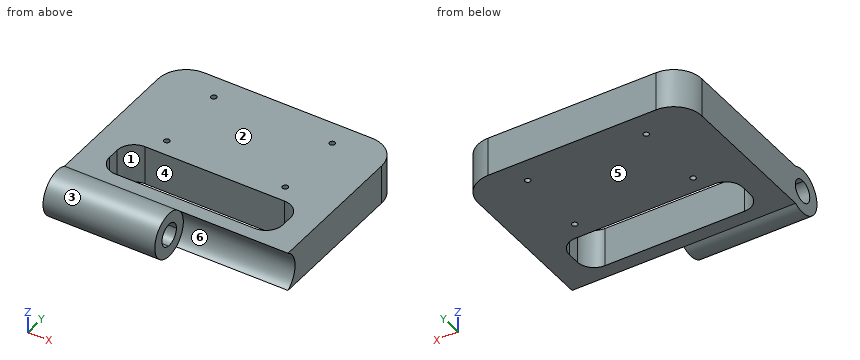
```python
from build123d import *

# Parameters (mm, degrees)
SKETCH1_W                = 40
SKETCH1_H                = 33.082043622
BOSS_EXTRUDE1_DEPTH      = 7
SKETCH2_R                = 4.1
CUT_EXTRUDE1_DEPTH       = 20
BOSS_EXTRUDE2_DEPTH      = 11
BOSS_EXTRUDE2_DEPTH_BACK = 9
SKETCH3_R                = 4
SKETCH3_R_2              = 2
FILLET1_R                = 5
SKETCH4_R                = 0.5
SKETCH4_W                = 31
SKETCH4_H                = 8.146627971
CUT_EXTRUDE2_DEPTH       = 45.095541639
FILLET2_R                = 3
SKETCH5_R                = 2
CUT_EXTRUDE3_DEPTH       = 56.229329833


with BuildPart() as part:
    # Sketch1 → Boss-Extrude1 (new body)
    with BuildSketch(Plane.XY):
        with Locations((-2.229213179, -16.994598242)):
            Rectangle(SKETCH1_W, SKETCH1_H)
    extrude(amount=BOSS_EXTRUDE1_DEPTH)

    # Sketch2 → Cut-Extrude1 (cut)
    with BuildSketch(Plane(origin=(17.770786821, 0, 0), x_dir=(0, 0, -1), z_dir=(1, 0, 0))):
        with Locations((-3.5, -33.535620053)):
            Circle(SKETCH2_R)
    extrude(amount=-CUT_EXTRUDE1_DEPTH, mode=Mode.SUBTRACT)

    # Sketch3 → Boss-Extrude2 (add, two sides: drawn at the far end of the back side and taken through both)
    with BuildSketch(Plane(origin=(-13.229213179, 0, 0), x_dir=(0, 0, -1), z_dir=(1, 0, 0)).offset(-BOSS_EXTRUDE2_DEPTH_BACK)):
        with Locations((-3.5, -33.336696075)):
            Circle(SKETCH3_R)
        with Locations((-3.5, -33.336696075)):
            Circle(SKETCH3_R_2, mode=Mode.SUBTRACT)
    extrude(amount=BOSS_EXTRUDE2_DEPTH + BOSS_EXTRUDE2_DEPTH_BACK)

    # Fillet1
    fillet1_edges = [part.edges().sort_by_distance(p)[0] for p in [
        (-22.229213179, -0.453576431, 3.5),
        (17.770786821, -0.453576431, 3.5),
    ]]
    fillet(fillet1_edges, radius=FILLET1_R)

    # Sketch4 → Cut-Extrude2 (cut, through all)
    with BuildSketch(Plane(origin=(0, 0, 0), x_dir=(-1, 0, 0), z_dir=(0, 0, -1))):
        with Locations((-8.470786821, -4.753576431)):
            Circle(SKETCH4_R)
        with Locations((12.729213179, -4.753576431)):
            Circle(SKETCH4_R)
        with Locations((12.729213179, -17.753576431)):
            Circle(SKETCH4_R)
        with Locations((-8.470786821, -17.753576431)):
            Circle(SKETCH4_R)
        with Locations((2.229213179, -24.826890417)):
            Rectangle(SKETCH4_W, SKETCH4_H)
    extrude(amount=-CUT_EXTRUDE2_DEPTH, mode=Mode.SUBTRACT)

    # Fillet2
    fillet2_edges = [part.edges().sort_by_distance(p)[0] for p in [
        (-17.729213179, -20.753576431, 3.5),
        (-17.729213179, -28.900204402, 3.5),
        (13.270786821, -28.900204402, 3.5),
        (13.270786821, -20.753576431, 3.5),
    ]]
    fillet(fillet2_edges, radius=FILLET2_R)

    # Sketch5 → Cut-Extrude3 (cut, through all)
    with BuildSketch(Plane.ZY.offset(22.229213179)):
        with Locations(Location((3.5, -33.336696075, 0), (0, 0, 90))):
            Circle(SKETCH5_R)
    extrude(amount=-CUT_EXTRUDE3_DEPTH, mode=Mode.SUBTRACT)


solid = part.part
```
The model under review builds one solid part; all positions refer to its coordinate system, in mm. Face numbers are marked on the shaded views. A direction names the side the tool comes from. Give positions to 0.01 mm unless a question says otherwise; leave off trailing zeros. Order: outer loops, then holes, each group sorted by start corner. A loop starts at its lowest first (then second) coordinate and runs counter-clockwise, first axis right, second up. Notation, with made-up numbers: (85, 27.25) - (89, 27.25) arc R23 cw to (89, 60.25) - close; hole circle Ø3 at (7.25, 26). An arc over 180 degrees is marked (long way). Use CSV: the item, a comma, the result in double quotes. Start each with the question number.
Q1. Clearance check with flat-ended pins moving along their axes: pin 1 Ø4 at (x, y) = (10.5, -32.5) entering from -Z; pin 2 Ø1.5 at (x, y) = (8.5, -12) entering from +Z; pin 3 Ø2 at (x, z) = (-1, 3) entering from -Y. State where each tip first meets the part, or that it passes through.
Q2. Tool access review of the marked faces 4, 5 and 6: name each direction out of +Z, -Z, +X, -X, +Y, -Y from which nothing blocks a thin tool from reaching the whole face with its end or side.
Q3. To check wall thickness, follow line 1 along Y through (x, z) = (6, 3.75); line 2 along X through (y, z) = (-24, 3.75); line 3 along Y through (x, z) = (-3.5, 2). State the ranges of each line that lie inside material, in increasing order. Write a range as [from, to].
Q4. The part is to be moulded in two halves that separate along Y. For the marked faces 1, 2 and 3, say which applies: +Y half, -Y half, draft (parallel to the pull), parting line (faces both ways), or undercut.
Q5. We need section A-A, the plane x = 0. Write out the cut boundary in (y, z).
Q6. We need section D-D, the plane y = -6. Write out the cut boundary in (x, z), and give its area (3 significant figures).
Q7. We need section B-B, the plane z = 4.75. Write out the cut boundary in (x, y), and give its area (3 significant figures).
Q8. We need section C-C, the plane x = -11.5. Write out the cut boundary in (y, z), and give its area (3 significant figures).
Outcome:
1,pin 1,"stops at z = 0"
1,pin 2,"stops at z = 7"
1,pin 3,"stops at y = -29.72"
2,face 4,"+Z, -Z"
2,face 5,"-Z, +X, -X, +Y"
2,face 6,"+X, -Y"
3,line 1,"y = [-29.44, -28.9], [-20.75, -0.45]"
3,line 2,"x = [-22.23, -17.73], [13.27, 17.77]"
3,line 3,"y = [-37.04, -34.66], [-32.01, -28.9], [-20.75, -0.45]"
4,face 1,"undercut"
4,face 2,"draft"
4,face 3,"parting line"
5,outline,"(-31.4, 0) - (-28.9, 0) - (-28.9, 7) - (-31.4, 7) arc R4.1 cw to start; (-20.75, 0) - (-0.45, 0) - (-0.45, 7) - (-20.75, 7) - close"
6,outline,"(-22.23, 0) - (17.77, 0) - (17.77, 7) - (-22.23, 7) - close"
6,area,"280 mm^2"
7,outline,"(-22.23, -37.14) - (-2.23, -37.14) - (-2.23, -34.9) - (-22.23, -34.9) - close; (-22.23, -31.78) - (-2.23, -31.78) - (-2.23, -29.63) - (17.77, -29.63) - (17.77, -5.45) arc R5 ccw to (12.77, -0.45) - (-17.23, -0.45) arc R5 ccw to (-22.23, -5.45) - close; hole (-17.73, -25.9) arc R3 ccw to (-14.73, -28.9) - (10.27, -28.9) arc R3 ccw to (13.27, -25.9) - (13.27, -23.75) arc R3 ccw to (10.27, -20.75) - (-14.73, -20.75) arc R3 ccw to (-17.73, -23.75) - close; hole circle Ø1 at (-12.73, -17.75); hole circle Ø1 at (-12.73, -4.75); hole circle Ø1 at (8.47, -17.75); hole circle Ø1 at (8.47, -4.75)"
7,area,"996 mm^2"
8,outline,"(-31.4, 0) - (-28.9, 0) - (-28.9, 7) - (-31.4, 7) arc R4 ccw (long way) to start; (-20.75, 0) - (-0.45, 0) - (-0.45, 7) - (-20.75, 7) - close; hole circle Ø4 at (-33.34, 3.5)"
8,area,"187 mm^2"
